```python
from build123d import *

# Parameters (mm, degrees)
F0_W           = 96
F0_H           = 43
F1_DEPTH       = 3.5
F2_T1_DEPTH    = 119.8484800354
F4_DEPTH       = 42
F5_T1_DEPTH    = 122.0704317696
F7_D           = 7
F7_CBORE_D     = 13
F7_CBORE_DEPTH = 3.5
F8_DEPTH       = 39.5
F3_W           = 89
F3_H           = 2.5
F9_DEPTH       = 3
F10_W          = 7.5
F10_H          = 2.5
F11_DEPTH      = 34.5
F12_W          = 10
F12_H          = 35
F13_DEPTH      = 3.5
F14_R          = 3


# Not quite as in the source:
# - a fillet or chamfer that OpenCascade refuses, or shapes differently, is made with other operations: its cross-section is extruded or revolved along the edge and cut away or added


with BuildPart() as f1:
    # F0 (on Top) → F1 (new body)
    with BuildSketch(Plane.XY):
        Rectangle(F0_W, F0_H)
    extrude(amount=F1_DEPTH)

    # F2: fillet of radius 5 on 1 edges, made by hand

    # F2_s2 → F2_t1 (cut)
    with BuildSketch(Plane.YZ.offset(-59.9242400177)):
        with BuildLine():
            ThreePointArc((-21.5, 3.5), (-19.6883438845, 0.9688711259), (-16.7303039929, 0))
            Line((-16.7303039929, 0), (-21.5, 0))
            Line((-21.5, 0), (-21.5, 3.5))
        make_face()
    extrude(amount=F2_T1_DEPTH, mode=Mode.SUBTRACT)

    # F3 (on face) → F4 (join)
    with BuildSketch(Plane.XY.offset(3.5)):
        Polygon((-48, 1.5), (-48, -3.5), (48, -3.5), (48, 1.5), (44.5, 1.5), (-44.5, 1.5), align=None)
    extrude(amount=F4_DEPTH)

    # F5: chamfer of 2.4 x 5.0317046378 on 1 edges, made by hand

    # F5_s2 → F5_t1 (cut)
    with BuildSketch(Plane.YZ.offset(-61.0352158848)):
        Polygon((1.5, 43.1), (-3.5317046378, 45.5), (1.5, 45.5), align=None)
    extrude(amount=F5_T1_DEPTH, mode=Mode.SUBTRACT)

    # F7 (through all)
    with Locations(Plane(origin=(0, 1.5, 0), x_dir=(-1, 0, 0), z_dir=(0, 1, 0))):
        with Locations((-27, 29.5)):
            CounterBoreHole(F7_D / 2, F7_CBORE_D / 2, F7_CBORE_DEPTH)

    # F3 (on face) → F8 (join)
    with BuildSketch(Plane.XY.offset(3.5)):
        Polygon((44.5, 1.5), (48, 1.5), (48, 21.5), (44.5, 21.5), (44.5, 19), align=None)
        Polygon((-48, 21.5), (-48, 1.5), (-44.5, 1.5), (-44.5, 19), (-44.5, 21.5), align=None)
    extrude(amount=F8_DEPTH)

    # F3 (on face) → F9 (join)
    with BuildSketch(Plane.XY.offset(3.5)):
        with Locations((0, 20.25)):
            Rectangle(F3_W, F3_H)
    extrude(amount=F9_DEPTH)

    # F10 (on face) → F11 (join)
    with BuildSketch(Plane.XY.offset(6.5)):
        with Locations((40.75, 20.25)):
            Rectangle(F10_W, F10_H)
        with Locations((-40.75, 20.25)):
            Rectangle(F10_W, F10_H)
    extrude(amount=F11_DEPTH)

    # F12 (on face) → F13 (cut)
    with BuildSketch(Plane.YZ.offset(-44.5)):
        with Locations((12, 25.5)):
            Rectangle(F12_W, F12_H)
    extrude(amount=-F13_DEPTH, mode=Mode.SUBTRACT)

    # F14
    f14_edges = [f1.edges().sort_by_distance(p)[0] for p in [
        (-48, 21.5, 21.5),
        (48, 21.5, 21.5),
        (-48, -19.688344, 0.968871),
        (48, -19.688344, 0.968871),
        (0, 21.5, 0),
        (48, 2.384848, 0),
        (-48, 2.384848, 0),
    ]]
    fillet(f14_edges, radius=F14_R)


solid = f1.part
```
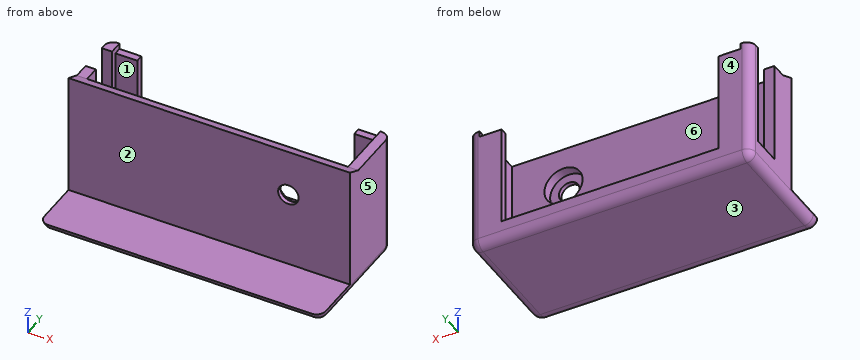
Build history of the part. All positions in model axes, mm. Face numbers are marked on the shaded views. A direction names the side the tool comes from. Round coordinates to 2 decimals unless told otherwise and drop trailing zeros. Loops run counter-clockwise (first coordinate to the right, second up) from the corner with the lowest first, then second, coordinate; pieces in that order, holes last. Notation, with made-up numbers: M 73.25,67.5 L 80.25,67.5 A32 ccw 80.25,104.5 Z; hole C -19.5,-12 d1. An arc over 180 degrees is marked long. Answer as CSV lines item,"result".
1. Cut at B-B on z = 29.5. Write the cut outline in (x, y), then the cut area to 3 significant figures.
Resolved:
outline,"M -48,-3.5 L 23.5,-3.5 L 23.5,-2 L 20.5,-2 L 20.5,1.5 L -44.5,1.5 L -44.5,7 L -48,7 Z; M -48,17 L -44.5,17 L -44.5,19 L -37,19 L -37,21.5 L -45,21.5 A3 ccw -48,18.5 Z; M 30.5,-3.5 L 48,-3.5 L 48,18.5 A3 ccw 45,21.5 L 37,21.5 L 37,19 L 44.5,19 L 44.5,1.5 L 33.5,1.5 L 33.5,-2 L 30.5,-2 Z"
area,"563 mm²"
2. Cut at C-C on x = 25. Write the cut outline in (y, z), then the cut area to 3 significant figures.
Resolved:
outline,"M -21.5,3.5 A5 ccw -16.73,0 L 18.5,0 A3 ccw 21.5,3 L 21.5,6.5 L 19,6.5 L 19,3.5 L 1.5,3.5 L 1.5,23.32 L -2,23.32 L -2,26.63 L -3.5,26.63 L -3.5,3.5 Z; M -3.5,32.37 L -2,32.37 L -2,35.68 L 1.5,35.68 L 1.5,43.1 L -3.5,45.48 Z"
area,"304 mm²"
3. Wall check: probe 1 along Y at (x, z) = (41, 34.5); probe 2 along X at (y, z) = (3, 40.5); probe 3 along Z at (x, y) = (-24, 16). Give the ranges that are in metal, low to high. Write a range as [from, to].
Resolved:
probe 1,"y = [-3.5, 1.5], [19, 21.5]"
probe 2,"x = [-48, -44.5], [44.5, 48]"
probe 3,"z = [0, 3.5]"
4. Cut at A-A on z = 37. Write the cut outline in (x, y).
Resolved:
outline,"M -48,-3.5 L 48,-3.5 L 48,18.5 A3 ccw 45,21.5 L 37,21.5 L 37,19 L 44.5,19 L 44.5,1.5 L -44.5,1.5 L -44.5,7 L -48,7 Z; M -48,17 L -44.5,17 L -44.5,19 L -37,19 L -37,21.5 L -45,21.5 A3 ccw -48,18.5 Z"
5. Flat gauge pins, fed straight in: P1, Ø21, axis at x = 27, z = 29.5, coming from the -Y side; P2, Ø4, axis at y = -4, z = 19.5, coming from the -X side; P3, Ø1, axis at x = -24, z = 35.5, coming from the +Y side; P4, Ø3, axis at x = -47, y = 5.5, coming from the +Z side. Where does each tip first touch, or does it go through?
Resolved:
P1,"stops at y = -3.5"
P2,"stops at x = -48"
P3,"stops at y = 1.5"
P4,"stops at z = 43"
6. Two-plate mould, pull along X, no slides. Class the marked faces 4, 5 and 6: released by +X, released by -X, zero draft, split by the parting line, or undercut.
Resolved:
face 4,"zero draft"
face 5,"released by +X"
face 6,"undercut"
7. 3-axis set-ups, long thin cutter, end or side, ignore diameter. For the marked faces 1, 2 and 3: which of +Z, -Z, +X, -X, +Y, -Y reach the whole face in a straight line?
Resolved:
face 1,"+Z"
face 2,"+Z, +X, -X, -Y"
face 3,"-Z, +X, -X, +Y, -Y"
8. Cut at D-D on y = 4.5. Write the cut outline in (x, z), then the cut area to 3 significant figures.
Resolved:
outline,"M -48,3 A3 ccw -45,0 L 45,0 A3 ccw 48,3 L 48,43 L 44.5,43 L 44.5,3.5 L -44.5,3.5 L -44.5,43 L -48,43 Z"
area,"609 mm²"
